Geometry: final body of the model. Coordinates: model frame, mm. A direction names the side the tool comes from. Give positions to 0.01 mm unless a question says otherwise; leave off trailing zeros. Loops run counter-clockwise (first coordinate to the right, second up) from the corner with the lowest first, then second, coordinate; pieces in that order, holes last. Notation, with made-up numbers: (48, 25) -> (68, 25) arc R21 ccw to (68, 39) -> close; hole circle Ø6 at (2.5, -14). An arc over 180 degrees is marked (long way). Answer in a Markdown table with one row per item. Add a question column.
1) Section query B-B (x = 7). Return the cut outline in (y, z).
2) Line query: line 1 (Y direction, x = 8, z = 1.3); line 2 (Z direction, x = -12, y = -28.7); line 3 (Z direction, x = -12, y = -9). Output: solid intervals per line, ascending. Write a range as from..to.
3) First-contact query: P1, Ø2, axis at x = -12, y = 24, coming from the -Z side; P2, Ø2, axis at y = -16, z = 1, coming from the -X side; P3, Ø3, axis at x = -12, z = 3, coming from the -Y side. Flat tips, straight axial feed; report the tip coordinate or a pass-through.
4) Draft query along Y for faces 1 (the flat face through (-12, 9, 5)), 2 (the cylindrical face through (-14.14, 0.42, 5.1)), 3 (the flat face through (-12, -26, 4)). Return one class per face: +Y half, -Y half, draft (parallel to the pull), parting line (faces both ways), or undercut.
5) Access query for faces 4 (the cylindrical face through (-12.31, -28.03, 5.38)), 5 (the flat face through (1, 0, 6)), 6 (the flat face through (7, 13, 3)). Directions: +Z, -Z, +X, -X, +Y, -Y. A direction counts if a zero-diameter tool reaches every point of the face in a straight line with its end or side. Return the directions, or none.
6) Section query A-A (y = 18.5). Give the number of separate pieces and of enclosed holes in the cut face, plus the area to 3 significant figures.
Autodesk Inventor part; units mm, degrees
ref_plane "YZ Plane" through (0, 0, 0) normal (1, 0, 0) x (0, 1, 0)
ref_plane "XZ Plane" through (0, 0, 0) normal (0, 1, 0) x (-1, 0, 0)
ref_plane "XY Plane" through (0, 0, 0) normal (0, 0, 1) x (1, 0, 0)
sketch "Náčrt1" plane through (0, 0, 0) normal (0, 0, 1) x (1, 0, 0)
  line L0 (-15, -30) -> (15, -30)
  line L1 (15, -30) -> (15, 30)
  line L2 (15, 30) -> (-15, 30)
  line L3 (-15, 30) -> (-15, -30)
  line L4 (-15, -30) -> (15, 30) construction
  line L5 (15, -30) -> (-15, 30) construction
  line L6 (0, 30) -> (0, 0)
  line L7 (-15, 15) -> (15, 15)
  line L8 (2, 17) -> (12, 17)
  line L9 (12, 17) -> (12, 24.5)
  line L10 (12, 24.5) -> (2, 24.5)
  line L11 (2, 24.5) -> (2, 17)
  line L12 (-2, 17) -> (-12, 17)
  line L13 (-12, 17) -> (-12, 24.5)
  line L14 (-12, 24.5) -> (-2, 24.5)
  line L15 (-2, 24.5) -> (-2, 17)
  line L16 (2, 13) -> (12, 13)
  line L17 (12, 13) -> (12, 5.5)
  line L18 (12, 5.5) -> (2, 5.5)
  line L19 (2, 5.5) -> (2, 13)
  line L20 (-12, 5.5) -> (-2, 5.5)
  line L21 (-12, 13) -> (-12, 5.5)
  line L22 (-2, 13) -> (-12, 13)
  line L23 (-2, 5.5) -> (-2, 13)
  dimension "d0" = 30
  dimension "d1" = 60
  dimension "d2" = 15
  dimension "d3" = 10
  dimension "d4" = 7.5
  dimension "d5" = 2
  dimension "d6" = 2
extrude "Vysunutí1" add sketch "Náčrt1" along normal blind 6
sketch "Náčrt2" plane through (15, -30, 0) normal (0, -1, 0) x (1, 0, 0)
  circle A0 centre (-27, 3) radius 2.4
  line L0 (-30, 0) -> (-30, 6)
  line L1 (-30, 6) -> (0, 6)
  line L2 (-30, 0) -> (0, 0)
  line L3 (-27, 0) -> (-27, 6)
  point P0 (-15, 0)
  point P1 (-30, 2)
  point P2 (-30, 4)
  dimension "d13" = 4.8
  dimension "d14" = 3
  dimension "d15" = 3
  dimension "d16" = 3
extrude "Vysunutí2" cut sketch "Náčrt2" against normal blind 4 contours A0 L3 | L3 A0
full round fillet "Plné kulaté zaoblení1" first side at (0.6667, -18.1667, 6) centre faces at (-15, 10, 2) second side at (0.6667, -18.1667, 0)
sketch "Náčrt3" plane through (15, 30, 6) normal (0, 1, 0) x (1, 0, 0)
  arc A0 (-27, 6) -> (-27, 0) centre (-27, 3) ccw
  point P0 (-15, 6)
hole "Díra1" at (-12, 30, 3) direction (0, -1, 0) diameter 1 end through all
properties part number "dvere_3D tisk"
Evaluation:
| question | item | result |
|---|---|---|
| 1 | outline | (-30, 0) -> (5.5, 0) -> (5.5, 6) -> (-30, 6) -> close; (13, 0) -> (17, 0) -> (17, 6) -> (13, 6) -> close; (24.5, 0) -> (30, 0) -> (30, 6) -> (24.5, 6) -> close |
| 2 | line 1 | -30..5.5, 13..17, 24.5..30 |
| 2 | line 2 | 0..0.6, 5.4..6 |
| 2 | line 3 | 0..2.5, 3.5..6 |
| 3 | P1 | z = 0 |
| 3 | P2 | x = -14.83 |
| 3 | P3 | y = -26 |
| 4 | face 1 | undercut |
| 4 | face 2 | draft |
| 4 | face 3 | -Y half |
| 5 | face 4 | -Y |
| 5 | face 5 | +Z, +X, -X, +Y, -Y |
| 5 | face 6 | +Z, -Z |
| 6 | separate pieces | 3 |
| 6 | enclosed holes | 0 |
| 6 | area | 55.7 mm² |
